Answer from the drawing. Dimensions are ordinates in mm from the lowest x, y and z of the part. A direction names the side the tool comes from. Round coordinates to 2 decimals unless told otherwise and drop trailing zeros. Write each loop counter-clockwise with the first axis right and the second up, starting at its lowest first coordinate (ties: lowest second). Pieces come first, ordered by that corner, then holes.
1. Straight lines are drawn through the part: probe 1 along X at (y, z) = (143, 49); probe 2 along Y at (x, z) = (191.5, 4); probe 3 along Z at (x, y) = (26.5, 57.5). For each, find the intervals that lie inside material, in ascending order.
2. Find section A-A (x = 69). Write down the section's boundary in (y, z), and give its area (3 significant figures).
3. Find section B-B (z = 44). Write down the section's boundary in (x, y), and give its area (3 significant figures).
4. Find section C-C (y = 74.5). Write down the section's boundary in (x, z).
5. A tool of negligible diameter and unlimited length cuts with its end or side. For the marked faces 1 and 2, from which of +Z, -Z, +X, -X, +Y, -Y can it reach the whole face along a straight path? Write none if from no direction.
6. Flat-ended cylindrical pins translate along their axes: pin 1 Ø1 at (x, z) = (99.5, 8) entering from -Y; pin 2 Ø4 at (x, y) = (133, 41) entering from +Z. Find the tip coordinate at first contact, or state that the pin passes through.
7. Determine the mould class of the marked faces 3, 4 and 5 for opening direction X: pulls with the +X half, pulls with the -X half, needs draft (parallel to the pull), parting line crosses it, or undercut.
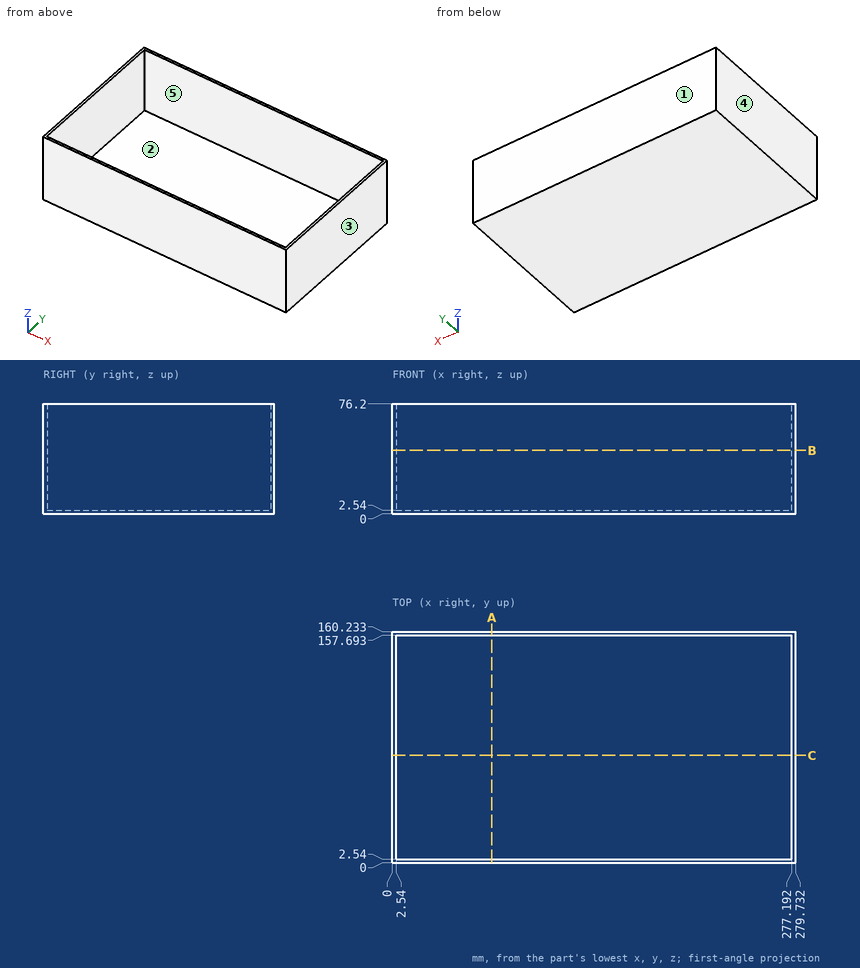
Worked answers:
1. probe 1: x = 0 to 2.54, 277.19 to 279.73
1. probe 2: y = 0 to 2.54, 157.69 to 160.23
1. probe 3: z = 0 to 2.54
2. outline: (0, 0) - (160.23, 0) - (160.23, 76.2) - (157.69, 76.2) - (157.69, 2.54) - (2.54, 2.54) - (2.54, 76.2) - (0, 76.2) - close
2. area: 781 mm2
3. outline: (0, 0) - (279.73, 0) - (279.73, 160.23) - (0, 160.23) - close; hole (2.54, 2.54) - (277.19, 2.54) - (277.19, 157.69) - (2.54, 157.69) - close
3. area: 2,210 mm2
4. outline: (0, 0) - (279.73, 0) - (279.73, 76.2) - (277.19, 76.2) - (277.19, 2.54) - (2.54, 2.54) - (2.54, 76.2) - (0, 76.2) - close
5. face 1: +Z, -Z, +X, -X, +Y
5. face 2: +Z
6. pin 1: stops at y = 0
6. pin 2: stops at z = 2.54
7. face 3: pulls with the +X half
7. face 4: pulls with the -X half
7. face 5: undercut
